```python
from build123d import *

# Parameters (mm, degrees)
SKETCH1_W           = 84
SKETCH1_H           = 34
BOSS_EXTRUDE1_DEPTH = 6
CUT_EXTRUDE1_DEPTH  = 75.823124768
SKETCH3_W           = 30
SKETCH3_H           = 11
BOSS_EXTRUDE2_DEPTH = 10.7
HOLE1_D             = 3.4
HOLE2_D             = 46
HOLE3_D             = 4.4
HOLE4_D             = 4.4
HOLE5_D             = 4.4
HOLE6_D             = 4.4
HOLE7_D             = 4.4
HOLE8_D             = 4.4
HOLE9_D             = 4.4
HOLE10_D            = 4.4
HOLE11_D            = 4.4
HOLE12_D            = 4.4
HOLE13_D            = 8
HOLE13_DEPTH        = 34
RIB1_REACH          = 59.09
SKETCH30_WALL_W     = 140.135684292
SKETCH30_WALL_H     = 5


with BuildPart() as part:
    # Sketch1 → Boss-Extrude1 (new body)
    with BuildSketch(Plane(origin=(0, 0, -14.3), x_dir=(-1, 0, 0), z_dir=(0, 0, -1))):
        with Locations((26.5, 12.5)):
            Rectangle(SKETCH1_W, SKETCH1_H)
    extrude(amount=-BOSS_EXTRUDE1_DEPTH)

    # Sketch2 → Cut-Extrude1 (cut, through all)
    with BuildSketch(Plane.XY.offset(-8.3)):
        with BuildLine():
            Line((-68.5, 29.5), (-68.5, 6.5))
            ThreePointArc((-68.5, 6.5), (-58.507750115, 8.78394482), (-50.5, 15.182178937))
            Line((-50.5, 15.182178937), (-50.5, 29.5))
            Line((-50.5, 29.5), (-68.5, 29.5))
        make_face()
    extrude(amount=-CUT_EXTRUDE1_DEPTH, mode=Mode.SUBTRACT)

    # Sketch3 → Boss-Extrude2 (add)
    with BuildSketch(Plane(origin=(0, 0, -14.3), x_dir=(-1, 0, 0), z_dir=(0, 0, -1))):
        with Locations((26.5, 1)):
            Rectangle(SKETCH3_W, SKETCH3_H)
    extrude(amount=BOSS_EXTRUDE2_DEPTH)

    # Hole1 (through all)
    with Locations(Plane(origin=(0, 0, -14.3), x_dir=(-1, 0, 0), z_dir=(0, 0, -1))):
        with Locations((46, 24.5)):
            Hole(HOLE1_D / 2)

    # Hole2 (through all)
    with Locations(Plane(origin=(0, 0, -14.3), x_dir=(-1, 0, 0), z_dir=(0, 0, -1))):
        with Locations((-15.5, 29.5)):
            Hole(HOLE2_D / 2)

    # Hole3 (through all)
    with Locations(Plane(origin=(0, 0, -14.3), x_dir=(-1, 0, 0), z_dir=(0, 0, -1))):
        with Locations((16.5, 12.25)):
            Hole(HOLE3_D / 2)

    # Hole4 (through all)
    with Locations(Plane(origin=(0, 0, -14.3), x_dir=(-1, 0, 0), z_dir=(0, 0, -1))):
        with Locations((36.5, 12.25)):
            Hole(HOLE4_D / 2)

    # Hole5 (through all)
    with Locations(Plane(origin=(0, 0, -14.3), x_dir=(-1, 0, 0), z_dir=(0, 0, -1))):
        with Locations((36.5, 24.75)):
            Hole(HOLE5_D / 2)

    # Hole6 (through all)
    with Locations(Plane(origin=(0, 0, -14.3), x_dir=(-1, 0, 0), z_dir=(0, 0, -1))):
        with Locations((16.5, 24.75)):
            Hole(HOLE6_D / 2)

    # Hole7 (through all)
    with Locations(Plane(origin=(0, 0, -25), x_dir=(-1, 0, 0), z_dir=(0, 0, -1))):
        with Locations((36, 1)):
            Hole(HOLE7_D / 2)

    # Hole8 (through all)
    with Locations(Plane(origin=(0, 0, -14.3), x_dir=(-1, 0, 0), z_dir=(0, 0, -1))):
        with Locations((48, 0)):
            Hole(HOLE8_D / 2)

    # Hole9 (through all)
    with Locations(Plane(origin=(0, 0, -14.3), x_dir=(-1, 0, 0), z_dir=(0, 0, -1))):
        with Locations((63, 0)):
            Hole(HOLE9_D / 2)

    # Hole10 (through all)
    with Locations(Plane.XY.offset(-8.3)):
        with Locations((-17, 1)):
            Hole(HOLE10_D / 2)

    # Hole11 (through all)
    with Locations(Plane(origin=(0, 0, -14.3), x_dir=(-1, 0, 0), z_dir=(0, 0, -1))):
        with Locations((5, 0)):
            Hole(HOLE11_D / 2)

    # Hole12 (through all)
    with Locations(Plane(origin=(0, 0, -14.3), x_dir=(-1, 0, 0), z_dir=(0, 0, -1))):
        with Locations((-10, 0)):
            Hole(HOLE12_D / 2)

    # Hole13
    with Locations(Plane.XZ.offset(4.5)):
        with Locations((-26.5, -25)):
            Hole(HOLE13_D / 2, depth=HOLE13_DEPTH)

    # Sketch30 wall → Rib1 (add, up to next)
    with BuildSketch(Plane(origin=(-26.5, 18, -17.65), x_dir=(0, -0.960093451224, -0.279679396661), z_dir=(0, -0.279679396661, 0.960093451224)), mode=Mode.PRIVATE) as rib1_sk1:
        Rectangle(SKETCH30_WALL_W, SKETCH30_WALL_H)
    rib1_tool1 = extrude(rib1_sk1.sketch, amount=RIB1_REACH, mode=Mode.PRIVATE) - part.part
    add(rib1_tool1.solids().sort_by_distance((-26.5, 18, -17.65))[0])


solid = part.part
```
Build history of the part. All positions in model axes, mm. A direction names the side the tool comes from. Round coordinates to 2 decimals unless told otherwise and drop trailing zeros. Write each loop counter-clockwise with the first axis right and the second up, starting at its lowest first coordinate (ties: lowest second). Pieces come first, ordered by that corner, then holes. Notation, with made-up numbers: (42, -27) - (68, -27) arc R27 cw to (68, 6) - close; hole circle Ø4 at (-28.75, -7.75). An arc over 180 degrees is marked (long way). Write each question's results on one line, items separated by ' | '. Start each with the question number.
Item 1: Saw through at B-B (x = -36.5). Write the cut outline in (y, z), and give its area (3 significant figures).
Item 2: Drop flat-ended pins along their axis: P1, Ø1.8, axis at y = 25.5, z = -11.5, coming from the -X side; P2, Ø12, axis at x = -21.5, y = 22.5, coming from the -Z side; P3, Ø5.5, axis at x = -16.5, y = 12.25, coming from the -Z side; P4, Ø1.5, axis at y = 26, z = -18, coming from the +X side. Give the stop position or say it passes through.
Item 3: Mould opens along Y. For faces 6 (the face through (-50.198, 0.097, -11.258)), 7 (the face through (-26.465, 18.161, -17.603)), 8 (the face through (-15.48, 22.8, -11.26)), 9 (the face through (-41.5, 1, -20)) say: pulls with the +Y half, pulls with the -Y half, needs draft (parallel to the pull), parting line crosses it, or undercut.
Item 4: Saw through at A-A (z = -23.25). Write the cut outline in (x, y), and give its area (3 significant figures).
Item 5: Wall check: L1, parallel to Y at x = -36, z = -12; L2, parallel to X at y = 24, z = -9.75; L3, parallel to X at y = 2, z = -22.25. Give the ranges that are in metal, low to high. Write a range as [from, to].
Item 6: Which spindle directions (+Z, -Z, +X, -X, +Y, -Y) get a long thin tool onto all of the face, cutting with end or side? Do faces 1 (the face through (-60.968, -0.843, -11.258)), 2 (the face through (-24, 15, -17)), 3 (the face through (-26, -4.5, -15)), 4 (the face through (-50.5, 22, -11)), 5 (the face through (-11.5, 1, -20)). Say none if no direction does.
Item 7: Saw through at C-C (y = 0). State how many separate pieces and enclosed holes the cut face has, and give its area (3 significant figures).
Results are:
1) outline: (-4.5, -25) - (-1.14, -25) - (-1.14, -8.3) - (-4.5, -8.3) - close; (3.14, -25) - (6.5, -25) - (6.5, -14.3) - (10.05, -14.3) - (10.05, -8.3) - (3.14, -8.3) - close; (14.45, -14.3) - (22.55, -14.3) - (22.55, -8.3) - (14.45, -8.3) - close; (26.95, -14.3) - (29.5, -14.3) - (29.5, -8.3) - (26.95, -8.3) - close | area: 197 mm²
2) P1: stops at x = -50.5 | P2: stops at z = -17.93 | P3: stops at z = -14.3 | P4: passes through
3) face 6: undercut | face 7: pulls with the +Y half | face 8: undercut | face 9: needs draft
4) outline: (-41.5, -4.5) - (-30.1, -4.5) - (-30.1, 6.5) - (-41.5, 6.5) - close; (-22.9, -4.5) - (-11.5, -4.5) - (-11.5, 6.5) - (-22.9, 6.5) - close; hole circle Ø4.4 at (-36, 1); hole circle Ø4.4 at (-17, 1) | area: 220 mm²
5) L1: y = [-4.5, -1.2], [3.2, 10.11], [14.39, 22.61], [26.89, 29.5] | L2: x = [-50.5, -47.62], [-44.38, -38.57], [-34.43, -18.57], [-14.43, -6.83] | L3: x = [-41.5, -37.96], [-34.04, -29.4], [-23.6, -18.96], [-15.04, -11.5]
6) face 1: +Z, -Z | face 2: -Z, +X, +Y | face 3: +Z, -Z, +X, -X, -Y | face 4: +Z, -Z, -X, +Y | face 5: -Z, +X, +Y, -Y
7) separate pieces: 7 | enclosed holes: 0 | area: 563 mm²
